Work out the finished part from the listing and answer in its coordinate system (mm). A direction names the side the tool comes from. Coordinates: 2 decimals unless noted, no trailing zeros. Order: outer loops, then holes, each group sorted by start corner. A loop starts at its lowest first (then second) coordinate and runs counter-clockwise, first axis right, second up. Notation, with made-up numbers: (29.25, 86.25) - (35.25, 86.25) arc R9 cw to (35.25, 101.25) - close; hole circle Ø5 at (-23.5, -3). An arc over 180 degrees is marked (long way). Answer as a JSON object with one key per item and string values. Group by question number.
1) Section C-C (y = 9.25) is taken. Give the vertices of the cut face in (x, z), plus the area to 3 significant figures.
2) The mould has two halves that part along X. Classify faces 1 (the face through (0, 9.75, 0)), 2 (the face through (-0.54, 9.49, 2.44)), 3 (the face through (0, 9, 2)): released by +X, released by -X, zero draft, split by the parting line, or undercut.
3) Each of these flat-tipped pins is pushed along its axis until it touches: P1, Ø0.8, axis at y = 10, z = 0.5, coming from the +X side; P2, Ø3, axis at x = -0.5, y = 3, coming from the -Z side; P3, Ø1, axis at x = -0.5, y = 5, coming from the +Z side. Where does it stop, or does it pass through?
4) Section A-A (z = 0) is taken. Give the vertices of the cut face in (x, y), plus the area to 3 significant figures.
5) Section D-D (y = 5) is taken. Give the vertices of the cut face in (x, z), plus the area to 3 significant figures.
6) A tool of negligible diameter and unlimited length cuts with its end or side. For faces 4 (the face through (-1.5, 4.44, -0.07)), 5 (the face through (0, 0, 0)), from which of +Z, -Z, +X, -X, +Y, -Y can it reach the whole face along a straight path? Write none if from no direction.
7) Find the intervals of material crossed by line 1 along Z through (x, y) = (-0.45, 4.75); line 2 along X through (y, z) = (5.75, -1.3); line 3 along X through (y, z) = (3, 0.15), in increasing order.
8) Section B-B (x = 0) is taken. Give the vertices of the cut face in (y, z).
from build123d import *

# Parameters (mm, degrees)
SKETCH1_R           = 1.5
BOSS_EXTRUDE1_DEPTH = 9
SKETCH2_R           = 2.5
BOSS_EXTRUDE2_DEPTH = 1
DOME1_FACE_RADIUS   = 2.5
DOME1_HEIGHT        = 0.5
SKETCH3_W           = 1.125
SKETCH3_H           = 0.75
SKETCH3_W_2         = 0.75
SKETCH3_H_2         = 1.125
CUT_EXTRUDE1_DEPTH  = 0.75


with BuildPart() as part:
    # Sketch1 → Boss-Extrude1 (new body)
    with BuildSketch(Plane(origin=(0, 0, 0), x_dir=(1, 0, 0), z_dir=(0, 1, 0))):
        Circle(SKETCH1_R)
    extrude(amount=BOSS_EXTRUDE1_DEPTH)

    # Sketch2 → Boss-Extrude2 (add)
    with BuildSketch(Plane(origin=(0, 9, 0), x_dir=(1, 0, 0), z_dir=(0, 1, 0))):
        Circle(SKETCH2_R)
    extrude(amount=BOSS_EXTRUDE2_DEPTH)

    # Dome1: a dome of height H over a round flat face of radius A is a cap of a sphere of radius (A * A + H * H) / (2 * H)
    dome1_r = (DOME1_FACE_RADIUS * DOME1_FACE_RADIUS + DOME1_HEIGHT * DOME1_HEIGHT) / (2 * DOME1_HEIGHT)
    dome1_base = Plane((0, 10, 0), z_dir=(0, 1, 0))
    with Locations(dome1_base.offset(DOME1_HEIGHT - dome1_r)):
        dome1_ball = Sphere(dome1_r, mode=Mode.PRIVATE)
    add(split(dome1_ball, bisect_by=dome1_base, keep=Keep.TOP, mode=Mode.PRIVATE))

    # Sketch3 → Cut-Extrude1 (cut)
    with BuildSketch(Plane(origin=(0, 10.5, 0), x_dir=(1, 0, 0), z_dir=(0, 1, 0))):
        with Locations((-0.9375, 0)):
            Rectangle(SKETCH3_W, SKETCH3_H)
        Rectangle(SKETCH3_W_2, SKETCH3_H)
        with Locations((0, 0.9375)):
            Rectangle(SKETCH3_W_2, SKETCH3_H_2)
        with Locations((0.9375, 0)):
            Rectangle(SKETCH3_W, SKETCH3_H)
        with Locations((0, -0.9375)):
            Rectangle(SKETCH3_W_2, SKETCH3_H_2)
    extrude(amount=-CUT_EXTRUDE1_DEPTH, mode=Mode.SUBTRACT)


solid = part.part
Report:
{
 "1": {"outline": "circle Ø5 at (0, 0)", "area": "19.6 mm²"},
 "2": {"face 1": "undercut", "face 2": "split by the parting line", "face 3": "zero draft"},
 "3": {"P1": "stops at x = 2.5", "P2": "stops at z = -1.5", "P3": "stops at z = 1.5"},
 "4": {"outline": "(-2.5, 9) - (-1.5, 9) - (-1.5, 0) - (1.5, 0) - (1.5, 9) - (2.5, 9) - (2.5, 10) arc R6.5 ccw to (1.5, 10.32) - (1.5, 9.75) - (-1.5, 9.75) - (-1.5, 10.32) arc R6.5 ccw to (-2.5, 10) - close", "area": "31.6 mm²"},
 "5": {"outline": "circle Ø3 at (0, 0)", "area": "7.07 mm²"},
 "6": {"face 4": "-Y", "face 5": "+Z, -Z, +X, -X, -Y"},
 "7": {"line 1": "z = -1.43 to 1.43", "line 2": "x = -0.75 to 0.75", "line 3": "x = -1.49 to 1.49"},
 "8": {"outline": "(0, -1.5) - (9, -1.5) - (9, -2.5) - (10, -2.5) arc R6.5 ccw to (10.32, -1.5) - (9.75, -1.5) - (9.75, 1.5) - (10.32, 1.5) arc R6.5 ccw to (10, 2.5) - (9, 2.5) - (9, 1.5) - (0, 1.5) - close"}
}
